Autodesk Inventor part; units mm, degrees
ref_plane "YZ Plane" through (0, 0, 0) normal (1, 0, 0) x (0, 1, 0)
ref_plane "XZ Plane" through (0, 0, 0) normal (0, 1, 0) x (-1, 0, 0)
ref_plane "XY Plane" through (0, 0, 0) normal (0, 0, 1) x (1, 0, 0)
sketch "Sketch1" plane through (0, 0, 0) normal (0, 1, 0) x (-1, 0, 0)
  line L0 (0, 0) -> (140, 0) construction
  line L1 (140, 0) -> (140, -290) construction
  line L2 (140, -290) -> (0, -290) construction
  line L3 (0, -290) -> (0, 0) construction
  line L4 (0, 0) -> (140, -290) construction
  line L5 (11.1043, 0) -> (140, -266.9982) construction
  line L6 (0, -23.0018) -> (128.8957, -290) construction
  line L7 (-10, -2.2875) -> (-10, 0)
  line L8 (140, 0) -> (0, -290) construction
  line L9 (140, -23.0018) -> (11.1043, -290) construction
  line L10 (128.8957, 0) -> (0, -266.9982) construction
  line L11 (150, -2.2875) -> (150, 0)
  line L12 (0, -23.0018) -> (0, 0)
  line L13 (140, -23.0018) -> (140, 0)
  line L14 (140, -266.9982) -> (140, -290)
  line L15 (0, -266.9982) -> (0, -290)
  line L16 (76.5, -105) -> (63.5, -105) construction
  line L17 (63.5, -105) -> (63.5, -185) construction
  line L18 (63.5, -185) -> (76.5, -185) construction
  line L19 (76.5, -185) -> (76.5, -105) construction
  line L20 (101.2667, -80.2333) -> (38.7333, -80.2333) construction
  line L21 (38.7333, -80.2333) -> (38.7333, -209.7667) construction
  line L22 (38.7333, -209.7667) -> (101.2667, -209.7667) construction
  line L23 (101.2667, -209.7667) -> (101.2667, -80.2333) construction
  line L24 (0, -23.0018) -> (38.7333, -103.2351)
  line L25 (38.7333, -186.7649) -> (0, -266.9982)
  line L26 (0, -290) -> (11.1043, -290)
  line L27 (49.8376, -209.7667) -> (90.1624, -209.7667)
  line L28 (49.8376, -209.7667) -> (11.1043, -290)
  line L29 (38.7333, -103.2351) -> (38.7333, -186.7649)
  line L30 (90.1624, -209.7667) -> (128.8957, -290)
  line L31 (128.8957, -290) -> (140, -290)
  line L32 (140, -266.9982) -> (101.2667, -186.7649)
  line L33 (101.2667, -186.7649) -> (101.2667, -103.2351)
  line L34 (101.2667, -103.2351) -> (140, -23.0018)
  line L35 (128.8957, 0) -> (90.1624, -80.2333)
  line L36 (90.1624, -80.2333) -> (49.8376, -80.2333)
  line L37 (49.8376, -80.2333) -> (11.1043, 0)
  line L38 (11.1043, 0) -> (0, 0)
  line L39 (128.8957, 0) -> (140, 0)
  line L40 (63.5, -105) -> (76.5, -105)
  line L41 (76.5, -185) -> (63.5, -185)
  line L42 (63.5, -105) -> (63.5, -185)
  line L43 (76.5, -185) -> (76.5, -105)
  point P0 (70, -105)
  point P1 (70, 0)
  point P2 (140, -145)
  point P3 (76.5, -145)
  dimension "d0" = 140
  dimension "d1" = 290
  dimension "d2" = 10
  dimension "d3" = 10
  dimension "d4" = 10
  dimension "d5" = 10
  dimension "d6" = 13
  dimension "d7" = 80
extrude "Extrusion1" add sketch "Sketch1" along normal blind 13
fillet "Fillet1" radius 10 4 edges at (-140, 6.5, -290) (0, 6.5, -290) (0, 6.5, 0) (-140, 6.5, 0)
sketch "Sketch2" plane through (0, 13, 0) normal (0, 1, 0) x (1, 0, 0)
  circle A0 centre (-8, 275) radius 5
  line L0 (-10, 290) -> (-11.1043, 290)
  line L1 (0, 266.9982) -> (0, 280) construction
  line L2 (-70, 345.1807) -> (-70, -192.6697) construction
  line L3 (0, 10) -> (0, 23.0018) construction
  line L4 (-90.1624, 80.2333) -> (-49.8376, 80.2333) construction
  circle A1 centre (-132, 275) radius 5
  line L5 (-255.5862, 145) -> (85.936, 145)
  line L6 (-38.7333, 103.2351) -> (-38.7333, 186.7649) construction
  circle A2 centre (-8, 15) radius 5
  circle A3 centre (-132, 15) radius 5
  point P0 (0, 0)
  point P1 (-70, 80.2333)
  point P2 (-38.7333, 145)
  dimension "d11" = 10
  dimension "d12" = 15
  dimension "d13" = 8
  dimension "d14" = 537.8504
  dimension "d15" = 341.5222
extrude "Extrusion2" add sketch "Sketch2" along normal blind 5
properties part number "SoportePlaca" material "Rubber, Silicone"
Check sheet for the modelled part. Datum: model origin and axes. Units: mm. A direction names the side the tool comes from. Give positions to 0.01 mm unless a question says otherwise; leave off trailing zeros. Order: outer loops, then holes, each group sorted by start corner. A loop starts at its lowest first (then second) coordinate and runs counter-clockwise, first axis right, second up. Notation, with made-up numbers: M -21,-26 L -13,-26 A18 cw -13,5 Z; hole C 60,10 d11. An arc over 180 degrees is marked long. Answer in a Markdown table with one row per item.
1) Cross-section at C-C, the plane x = -20.5. Enter the section's corners in (y, z), plus the area to 3 significant figures.
Filled sheet:
| item | result |
|---|---|
| outline | M 0,-270.54 L 13,-270.54 L 13,-224.53 L 0,-224.53 Z; M 0,-65.47 L 13,-65.47 L 13,-19.46 L 0,-19.46 Z |
| area | 1,200 mm2 |
2) Thickness scan on L1, parallel to X at y = 10.5, z = -115; L2, parallel to X at y = 5, z = -36.5; L3, parallel to Y at x = -120, z = -231. Record the ranges inside material, lowest first. Write a range as [from, to].
Filled sheet:
| item | result |
|---|---|
| L1 | x = [-101.27, -76.5], [-63.5, -38.73] |
| L2 | x = [-133.48, -111.28], [-28.72, -6.52] |
| L3 | y = [0, 13] |
3) Access from +Z, -Z, +X, -X, +Y, -Y to the whole of each face (thin tool, end or side, straight path). Record for faces 5 (the flat face through (-38.733, 6, -144)), 6 (the flat face through (-30.742, 6.409, -249.322)), 7 (the cylindrical face through (-132.651, 15.465, -270.043)), 8 (the flat face through (-120.904, 6.409, -227.443)).
Filled sheet:
| item | result |
|---|---|
| face 5 | +X, +Y, -Y |
| face 6 | -Z, +Y, -Y |
| face 7 | +Y |
| face 8 | -X, +Y, -Y |
4) Cross-section at A-A, the plane y = 7.75. Enter the section's corners in (x, z), plus the area to 3 significant figures.
Filled sheet:
| item | result |
|---|---|
| outline | M -140,-280 A10 ccw -130,-290 L -128.9,-290 L -90.16,-209.77 L -49.84,-209.77 L -11.1,-290 L -10,-290 A10 ccw 0,-280 L 0,-267 L -38.73,-186.76 L -38.73,-103.24 L 0,-23 L 0,-10 A10 ccw -10,0 L -11.1,0 L -49.84,-80.23 L -90.16,-80.23 L -128.9,0 L -130,0 A10 ccw -140,-10 L -140,-23 L -101.27,-103.24 L -101.27,-186.76 L -140,-267 Z; hole M -76.5,-185 L -63.5,-185 L -63.5,-105 L -76.5,-105 Z |
| area | 14,100 mm2 |
5) Cross-section at D-D, the plane z = -275. Enter the section's corners in (x, y).
Filled sheet:
| item | result |
|---|---|
| outline | M -140,0 L -121.65,0 L -121.65,13 L -127,13 L -127,18 L -137,18 L -137,13 L -140,13 Z; M -18.35,0 L 0,0 L 0,13 L -3,13 L -3,18 L -13,18 L -13,13 L -18.35,13 Z |
6) Cross-section at B-B, the plane z = -181. Enter the section's corners in (x, y), plus the area to 3 significant figures.
Filled sheet:
| item | result |
|---|---|
| outline | M -101.27,0 L -76.5,0 L -76.5,13 L -101.27,13 Z; M -63.5,0 L -38.73,0 L -38.73,13 L -63.5,13 Z |
| area | 644 mm2 |
7) Gauge pin test, flat ends, axial feed: P1, Ø10, axis at y = 10.5, z = -202, coming from the +X side; P2, Ø6.5, axis at x = -79, y = 8, coming from the -Z side; P3, Ø4, axis at y = 12.5, z = -234, coming from the +X side. Record the tip position at first contact, or that the pin passes through.
Filled sheet:
| item | result |
|---|---|
| P1 | stops at x = -28.96 |
| P2 | stops at z = -209.77 |
| P3 | stops at x = -14.96 |
8) Release check for a two-part mould opening along Z. For faces 1 (the cylindrical face through (-129.693, 15.465, -19.436)), 2 (the flat face through (-19.638, 6.409, -226.32)), 3 (the cylindrical face through (-2.85, 6.59, -286.99)), 4 (the flat face through (-132, 18, -275)) record: +Z half, -Z half, draft (parallel to the pull), parting line (faces both ways), or undercut.
Filled sheet:
| item | result |
|---|---|
| face 1 | undercut |
| face 2 | undercut |
| face 3 | -Z half |
| face 4 | draft |
